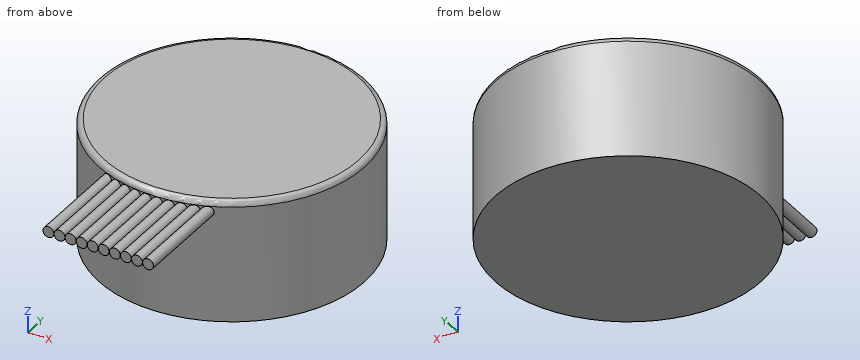
```python
from build123d import *

# Parameters (mm, degrees)
ESQUISSE1_R        = 12
BOSS_EXTRU_1_DEPTH = 11
CONG_1_R           = 0.5
ESQUISSE2_R        = 0.49
BOSS_EXTRU_2_DEPTH = 20


with BuildPart() as part:
    # Esquisse1 → Boss.-Extru.1 (new body)
    with BuildSketch(Plane.XY):
        Circle(ESQUISSE1_R)
    extrude(amount=BOSS_EXTRU_1_DEPTH)

    # Congé1
    cong_1_edges = [part.edges().sort_by_distance(p)[0] for p in [
        (-12, 0, 11),
    ]]
    fillet(cong_1_edges, radius=CONG_1_R)

    # Esquisse2 → Boss.-Extru.2 (add)
    with BuildSketch(Plane(origin=(0, 0, 0), x_dir=(1, 0, 0), z_dir=(0, 1, 0))):
        with Locations(Location((0.5, -10, 0), (0, 0, 270))):
            Circle(ESQUISSE2_R)
        with Locations(Location((1.5, -10, 0), (0, 0, 270))):
            Circle(ESQUISSE2_R)
        with Locations(Location((2.5, -10, 0), (0, 0, 270))):
            Circle(ESQUISSE2_R)
        with Locations(Location((3.5, -10, 0), (0, 0, 270))):
            Circle(ESQUISSE2_R)
        with Locations(Location((4.5, -10, 0), (0, 0, 270))):
            Circle(ESQUISSE2_R)
        with Locations(Location((-0.5, -10, 0), (0, 0, 270))):
            Circle(ESQUISSE2_R)
        with Locations(Location((-1.5, -10, 0), (0, 0, 270))):
            Circle(ESQUISSE2_R)
        with Locations(Location((-2.5, -10, 0), (0, 0, 270))):
            Circle(ESQUISSE2_R)
        with Locations(Location((-3.5, -10, 0), (0, 0, 270))):
            Circle(ESQUISSE2_R)
        with Locations(Location((-4.5, -10, 0), (0, 0, 270))):
            Circle(ESQUISSE2_R)
    extrude(amount=-BOSS_EXTRU_2_DEPTH)


solid = part.part
```
Geometry check sheet. Reference: the model listing, model coordinates, mm. Round coordinates to 2 decimals unless told otherwise and drop trailing zeros. Loops run counter-clockwise (first coordinate to the right, second up) from the corner with the lowest first, then second, coordinate; pieces in that order, holes last. Notation, with made-up numbers: (82.25, -27.5) - (86.25, -27.5) arc R28 ccw to (86.25, -4.5) - close; hole circle Ø11 at (57, 24.25). An arc over 180 degrees is marked (long way). Write each question's results on one line, items separated by ' | '. Start each with the question number.
Q1. Cross-section at A-A on z = 2.75. Enter the section's corners in (x, y).
Q2. Thickness scan on line 1 (Y direction, x = 9.5, z = 2.75); line 2 (X direction, y = -9, z = 10); line 3 (X direction, y = -6, z = 5.75). Record the ranges inside material, lowest first. Write a range as [from, to].
Q3. Gauge pin test, flat ends, axial feed: P1, Ø6, axis at x = 0, z = 5.5, coming from the -Y side; P2, Ø1.5, axis at y = -4, z = 1.5, coming from the +X side. Record the tip position at first contact, or that the pin passes through.
Answers below:
1) outline: circle Ø24 at (0, 0)
2) line 1: y = [-7.33, 7.33] | line 2: x = [-7.94, 7.94] | line 3: x = [-10.39, 10.39]
3) P1: stops at y = -12 | P2: stops at x = 11.55
